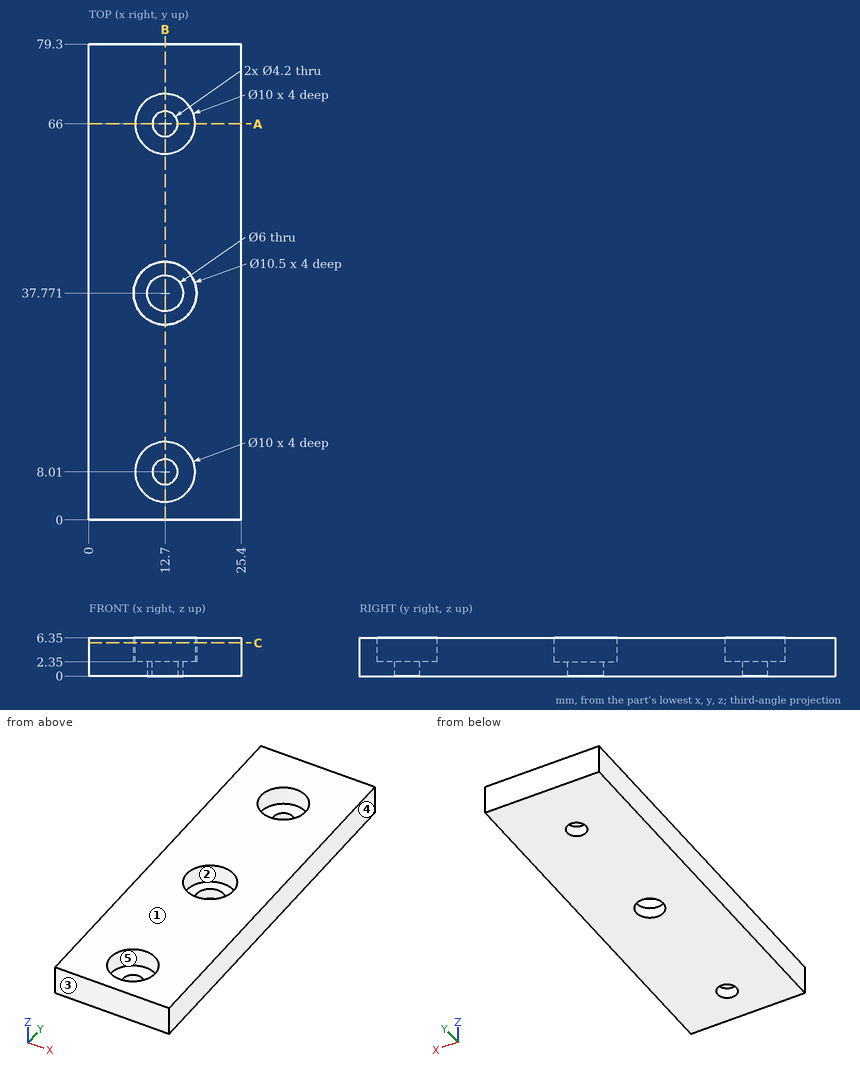
Study the drawing (mm; zero at the part's minimum x, y, z) and answer. A direction names the side the tool comes from. Coordinates: 2 decimals unless noted, no trailing zeros. Write each loop counter-clockwise with the first axis right and the second up, starting at its lowest first coordinate (ties: lowest second). Pieces come first, ordered by that corner, then holes.
Q1. A cutting plane is placed at B-B, the plane x = 12.7. Give the vertices of the cut face in (y, z), then the cut area to 3 significant figures.
Q2. Which of the six approach directions +Z, -Z, +X, -X, +Y, -Y give full straight-line access (tool end or side, diameter ignored) to the marked faces 4 and 5?
Q3. A cutting plane is placed at A-A, the plane y = 66. Give the vertices of the cut face in (x, z).
Q4. Determine the mould class of the marked faces 1, 2 and 3 for opening direction Y: released by +Y, released by -Y, zero draft, split by the parting line, or undercut.
Q5. A cutting plane is placed at C-C, the plane z = 5.5. Give the vertices of the cut face in (x, y), then the cut area to 3 significant figures.
Q6. Find the intervals of material crossed by line 1 (Y direction, x = 12.7, z = 1.65); line 2 (Y direction, x = 12.7, z = 3.95); line 3 (X direction, y = 8, z = 5.75), in increasing order.
Q7. This flat-tipped pin is pushed along its axis until it touches: pin 1 Ø3 at (x, y) = (15, 9.5) entering from +Z. Where does it stop, or does it pass through?
Findings below:
1. outline: (0, 0) - (5.91, 0) - (5.91, 2.35) - (3.01, 2.35) - (3.01, 6.35) - (0, 6.35) - close; (10.11, 0) - (34.77, 0) - (34.77, 2.35) - (32.52, 2.35) - (32.52, 6.35) - (13.01, 6.35) - (13.01, 2.35) - (10.11, 2.35) - close; (40.77, 0) - (63.9, 0) - (63.9, 2.35) - (61, 2.35) - (61, 6.35) - (43.02, 6.35) - (43.02, 2.35) - (40.77, 2.35) - close; (68.1, 0) - (79.3, 0) - (79.3, 6.35) - (71, 6.35) - (71, 2.35) - (68.1, 2.35) - close
1. area: 348 mm2
2. face 4: +Z, -Z, +X, +Y, -Y
2. face 5: +Z
3. outline: (0, 0) - (10.6, 0) - (10.6, 2.35) - (7.7, 2.35) - (7.7, 6.35) - (0, 6.35) - close; (14.8, 0) - (25.4, 0) - (25.4, 6.35) - (17.7, 6.35) - (17.7, 2.35) - (14.8, 2.35) - close
4. face 1: zero draft
4. face 2: undercut
4. face 3: released by -Y
5. outline: (0, 0) - (25.4, 0) - (25.4, 79.3) - (0, 79.3) - close; hole circle Ø10.5 at (12.7, 37.77); hole circle Ø10 at (12.7, 8.01); hole circle Ø10 at (12.7, 66)
5. area: 1,770 mm2
6. line 1: y = 0 to 5.91, 10.11 to 34.77, 40.77 to 63.9, 68.1 to 79.3
6. line 2: y = 0 to 3.01, 13.01 to 32.52, 43.02 to 61, 71 to 79.3
6. line 3: x = 0 to 7.7, 17.7 to 25.4
7. pin 1: stops at z = 2.35
